Source: CAD feature listing. Evaluate the final solid. Frame: model axes, mm. A direction names the side the tool comes from. Round coordinates to 2 decimals unless told otherwise and drop trailing zeros. Loops run counter-clockwise (first coordinate to the right, second up) from the corner with the lowest first, then second, coordinate; pieces in that order, holes last. Notation, with made-up numbers: (46.5, 79) - (104.5, 79) arc R23 cw to (104.5, 101) - close; hole circle Ø2 at (18, -8). An arc over 180 degrees is marked (long way). One line per question, with ' | ' between items.
from build123d import *

# Parameters (mm, degrees)
F0_R     = 1.625
F1_DEPTH = 6
F2_R     = 2.99999


# Not quite as in the source:
# - a fillet or chamfer is up to 0.001 mm smaller than in the source, because OpenCascade refuses the exact size


with BuildPart() as f1:
    # F0 (on Front) → F1 (new body)
    with BuildSketch(Plane.XZ):
        with BuildLine():
            Line((12.0862172917, 3.4724390134), (0.0079838936, 3.4999908939))
            ThreePointArc((0.0079838936, 3.4999908939), (0.0039919494, 3.4999977235), (0, 3.5))
            ThreePointArc((0, 3.5), (-2.4748737342, -2.4748737342), (3.5, 0))
            Line((3.5, 0), (12.3, 0))
            Line((12.3, 0), (10.9180201011, -2.9636654571))
            Line((10.9180201011, -2.9636654571), (18.0862172917, -2.9636654571))
            Line((18.0862172917, -2.9636654571), (18.0862172917, 12.0363345429))
            Line((18.0862172917, 12.0363345429), (12.0862172917, 12.0363345429))
            Line((12.0862172917, 12.0363345429), (12.0862172917, 3.4724390134))
        make_face()
        Circle(F0_R, mode=Mode.SUBTRACT)
    extrude(amount=F1_DEPTH)

    # F2 (radius 3 in the source; OpenCascade refuses exactly that, so slightly less here)
    f2_edges = [f1.edges().sort_by_distance(p)[0] for p in [
        (12.086217, -3, 12.036335),
        (12.086217, -3, 3.472439),
        (18.086217, -3, 12.036335),
        (18.086217, -3, -2.963665),
    ]]
    fillet(f2_edges, radius=F2_R)


solid = f1.part
1. Contact query for flat-ended pins moving along their axis: P1, Ø3, axis at x = 6.5, y = -2, coming from the -Z side; P2, Ø2, axis at x = 12.5, y = -3, coming from the +Z side; P3, Ø3.5, axis at x = 14, y = -3, coming from the -Z side. Output: stop coordinate, or through.
Worked out:
P1: stops at z = 0 | P2: stops at z = 11.58 | P3: stops at z = -2.96
2. Mould query, pull axis Z, two halves, no side actions, for faces 4 (the cylindrical face through (-1.29, -2.96, -0.99)), 5 (the flat face through (11.6, -3, -1.5)), 6 (the cylindrical face through (-2.555, -2.958, -2.392)), 7 (the cylindrical face through (11.18, -3.04, 4.33)). Classes: released by +Z, released by -Z, zero draft, split by the parting line, or undercut.
Worked out:
face 4: undercut | face 5: undercut | face 6: split by the parting line | face 7: released by +Z
3. Section query C-C, the plane x = 0.25. Return loops of the section in (y, z).
Worked out:
outline: (-6, -3.49) - (0, -3.49) - (0, -1.61) - (-6, -1.61) - close; (-6, 1.61) - (0, 1.61) - (0, 3.5) - (-6, 3.5) - close
4. Access query for faces 1 (the flat face through (13, -3, -2.964)), 2 (the flat face through (12.086, -3, 8)), 3 (the cylindrical face through (17.184, -3.042, 11.181)). Directions: +Z, -Z, +X, -X, +Y, -Y. A direction counts if a zero-diameter tool reaches every point of the face in a straight line with its end or side. Return the directions, or none.
Worked out:
face 1: -Z, +X, +Y, -Y | face 2: +Z, -X, +Y, -Y | face 3: +Z, +X, +Y, -Y
5. Section query B-B, the plane z = 0.75. Return loops of the section in (x, y), plus the area to 3 significant figures.
Worked out:
outline: (-3.42, -6) - (-1.44, -6) - (-1.44, 0) - (-3.42, 0) - close; (1.44, -6) - (18.09, -6) - (18.09, 0) - (1.44, 0) - close | area: 112 mm2
6. Material intervals for probe 1 along Z at (x, y) = (0, -3.05) (3 decimals); probe 2 along X at (y, z) = (-3, 8.5); probe 3 along Z at (x, y) = (8, -1.6), sorted ascending.
Worked out:
probe 1: z = -3.5 to -1.625, 1.625 to 3.5 | probe 2: x = 12.09 to 18.09 | probe 3: z = 0 to 3.48
7. Section query D-D, the plane z = 4.5. Return loops of the section in (x, y), plus the area to 3 significant figures.
Worked out:
outline: (11.34, -6) - (18.09, -6) - (18.09, 0) - (11.34, 0) - close | area: 40.5 mm2
